```python
from build123d import *

# Parameters (mm, degrees)
F1_DEPTH = 63.5
F2_DEPTH = 25.4
F3_DEPTH = 7.9375


with BuildPart() as f1:
    # F0 (on Front) → F1 (new body, symmetric)
    with BuildSketch(Plane.XZ):
        Polygon((22.225, 9.525), (-41.275, 9.525), (-41.275, -9.525), (41.275, -9.525), (41.275, 9.525), align=None)
    extrude(amount=F1_DEPTH, both=True)

    # F0 (on Front) → F2 (join, symmetric)
    with BuildSketch(Plane.XZ):
        with BuildLine():
            Line((22.225, 27.0002), (22.225, 9.525))
            Line((22.225, 9.525), (41.275, 9.525))
            Line((41.275, 9.525), (41.275, 27.0002))
            ThreePointArc((41.275, 27.0002), (45.92468, 38.22552), (57.15, 42.8752))
            Line((57.15, 42.8752), (60.325, 42.8752))
            Line((60.325, 42.8752), (60.325, 61.9252))
            Line((60.325, 61.9252), (57.15, 61.9252))
            add(Edge.make_bspline(
                [(56.101355, 61.909453), (56.450531, 61.915616), (56.800083, 61.920866), (57.15, 61.9252)],
                knots=[110.770194, 110.770194, 110.770194, 110.770194, 111.504536, 111.504536, 111.504536, 111.504536], degree=3))
            ThreePointArc((56.101355, 61.909453), (32.086286, 51.322327), (22.225, 27.0002))
        make_face()
        Polygon((85.725, 61.9252), (60.325, 61.9252), (60.325, 42.8752), (85.725, 42.8752), (85.725, 52.3875), align=None)
        Polygon((111.125, 61.9252), (85.725, 61.9252), (85.725, 52.3875), (85.725, 42.8752), (111.125, 42.8752), align=None)
    extrude(amount=F2_DEPTH, both=True)

    # F0 (on Front) → F3 (join, symmetric)
    with BuildSketch(Plane.XZ):
        with BuildLine():
            add(Edge.make_bspline(
                [(-41.275, 9.525), (-40.702354, 39.286222), (3.430554, 60.979856), (56.101355, 61.909453)],
                knots=[0, 0, 0, 0, 110.770194, 110.770194, 110.770194, 110.770194], degree=3))
            Line((-41.275, 9.525), (22.225, 9.525))
            Line((22.225, 9.525), (22.225, 27.0002))
            ThreePointArc((22.225, 27.0002), (32.086286, 51.322327), (56.101355, 61.909453))
        make_face()
    extrude(amount=F3_DEPTH, both=True)


solid = f1.part
```
CAD build for the part. Positions are in the model's coordinates, mm. A direction names the side the tool comes from. Give positions to 0.01 mm unless a question says otherwise; leave off trailing zeros. Order: outer loops, then holes, each group sorted by start corner. A loop starts at its lowest first (then second) coordinate and runs counter-clockwise, first axis right, second up. Notation, with made-up numbers: M -13,59 L 28,59 A19 cw 28,73 Z; hole C 79.5,31 d7. An arc over 180 degrees is marked long. Put each result on its own line as item: value. Start each with the question number.
(1) Mould opens along Y. For faces 1 (the flat face through (84, 0, 42.875)), 2 (the flat face through (56, 25.4, 48)), 3 (the flat face through (-3, -7.938, 30)) say: +Y half, -Y half, draft (parallel to the pull), parting line (faces both ways), or undercut.
(2) Drill centre lines: line 1 along Y through (x, z) = (32.5, 23); line 2 along X through (y, z) = (13, 6) (3 decimals); line 3 along Z through (x, y) = (-32, 32) (3 decimals). Where is each one in solid material? Low to high.
(3) Which spindle directions (+Z, -Z, +X, -X, +Y, -Y) get a long thin tool onto all of the face, cutting with end or side? Do faces 4 (the flat face through (41.275, -1, 4)), 5 (the flat face through (56, -25.4, 48)), 6 (the flat face through (22.225, -17, 18)). Say none if no direction does.
(4) Saw through at A-A, the plane z = 2.5. Write the cut outline in (x, y) (3 decimals).
(5) Saw through at B-B, the plane y = 49.5. Write the cut outline in (x, z) (3 decimals).
(6) Flat gauge pins, fed straight in: pin 1 Ø15.5 at (x, z) = (54.5, 43.5) entering from +Y; pin 2 Ø12 at (x, y) = (90, 25) entering from -Z; pin 3 Ø3 at (x, z) = (18, 29) entering from +Y; pin 4 Ø19 at (y, z) = (18.5, 15) entering from -X (3 decimals). Where does each tip first touch, or does it go through?
Check result:
1. face 1: draft
1. face 2: +Y half
1. face 3: -Y half
2. line 1: y = -25.4 to 25.4
2. line 2: x = -41.275 to 41.275
2. line 3: z = -9.525 to 9.525
3. face 4: -Z, +X, +Y, -Y
3. face 5: +Z, +X, -X, -Y
3. face 6: +Z, -X, -Y
4. outline: M -41.275,-63.5 L 41.275,-63.5 L 41.275,63.5 L -41.275,63.5 Z
5. outline: M -41.275,-9.525 L 41.275,-9.525 L 41.275,9.525 L -41.275,9.525 Z
6. pin 1: stops at y = 25.4
6. pin 2: stops at z = 42.88
6. pin 3: stops at y = 7.94
6. pin 4: stops at x = -41.275
